Work out the finished part from the listing and answer in its coordinate system (mm). Face numbers are marked on the shaded views. A direction names the side the tool comes from. Coordinates: 2 decimals unless noted, no trailing zeros. Order: outer loops, then holes, each group sorted by start corner. A loop starts at its lowest first (then second) coordinate and runs counter-clockwise, first axis right, second up. Notation, with made-up numbers: (29.25, -30) - (44.25, -30) arc R21 cw to (44.25, -7) - close; hole circle Ø7 at (36, 85.25). An arc over 180 degrees is marked (long way). Use CSV: the item, a comma, the result in double quotes. Start each with the question number.
from build123d import *

# Parameters (mm, degrees)
SKETCH1_R               = 6.5
BOSS_EXTRUDE1_DEPTH     = 17.5
SKETCH2_R               = 8.62249149
SKETCH2_R_2             = 5.56
CUT_EXTRUDE1_DEPTH      = 8
CUT_EXTRUDE2_DEPTH      = 20.767397401
CUT_EXTRUDE2_DEPTH_BACK = 20.767397401
SKETCH4_R               = 3
SKETCH5_R               = 8
SKETCH5_R_2             = 3.869185068
BOSS_EXTRUDE2_DEPTH     = 1
SKETCH6_R               = 8
SKETCH6_R_2             = 3
BOSS_EXTRUDE3_DEPTH     = 3.2


with BuildPart() as part:
    # Sketch1 → Boss-Extrude1 (new body)
    with BuildSketch(Plane(origin=(0, 0, 0), x_dir=(1, 0, 0), z_dir=(0, 1, 0))):
        with Locations(Location((0, 0, 0), (0, 0, 270))):
            Circle(SKETCH1_R)
    extrude(amount=BOSS_EXTRUDE1_DEPTH)

    # Sketch2 → Cut-Extrude1 (cut)
    with BuildSketch(Plane(origin=(0, 11.2, 0), x_dir=(1, 0, 0), z_dir=(0, 1, 0))):
        Circle(SKETCH2_R)
        with Locations(Location((0, 0, 0), (0, 0, 270))):
            Circle(SKETCH2_R_2, mode=Mode.SUBTRACT)
    extrude(amount=-CUT_EXTRUDE1_DEPTH, mode=Mode.SUBTRACT)

    # Sketch4 → Cut-Extrude2 (cut, two sides: drawn at the far end of the back side and taken through both)
    with BuildSketch(Plane(origin=(0, 17.5, 0), x_dir=(1, 0, 0), z_dir=(0, 1, 0)).offset(-CUT_EXTRUDE2_DEPTH_BACK)):
        with Locations(Location((0, 0, 0), (0, 0, 270))):
            Circle(SKETCH4_R)
    extrude(amount=CUT_EXTRUDE2_DEPTH + CUT_EXTRUDE2_DEPTH_BACK, mode=Mode.SUBTRACT)

    # Sketch5 → Boss-Extrude2 (add)
    with BuildSketch(Plane(origin=(0, 11.2, 0), x_dir=(1, 0, 0), z_dir=(0, 1, 0))):
        with Locations(Location((0, 0, 0), (0, 0, 270))):
            Circle(SKETCH5_R)
        Circle(SKETCH5_R_2, mode=Mode.SUBTRACT)
    extrude(amount=BOSS_EXTRUDE2_DEPTH)

    # Sketch6 → Boss-Extrude3 (add)
    with BuildSketch(Plane(origin=(0, 0, 0), x_dir=(1, 0, 0), z_dir=(0, 1, 0))):
        with Locations(Location((0, 0, 0), (0, 0, 270))):
            Circle(SKETCH6_R)
        with Locations(Location((0, 0, 0), (0, 0, 270))):
            Circle(SKETCH6_R_2, mode=Mode.SUBTRACT)
    extrude(amount=BOSS_EXTRUDE3_DEPTH)


solid = part.part
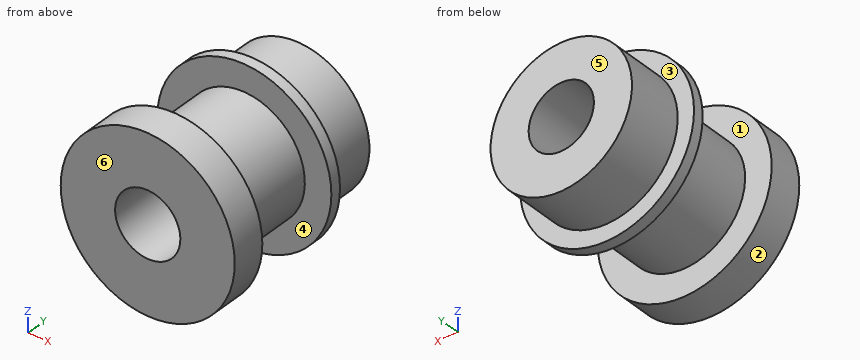
1) For a pull along Y with two mould halves and no side action, classify the marked faces 4, 5 and 6 as +Y half, -Y half, draft (parallel to the pull), parting line (faces both ways), or undercut.
2) The part is cut by section D-D on z = 3.5. Determine the outline of the cut face in (x, y), plus the area to 3 significant figures.
3) The part is cut by section A-A on x = 0. Determine the outline of the cut face in (y, z), plus the area to 3 significant figures.
4) Flat-ended cylindrical pins translate along their axes: P1, Ø6, axis at x = 5, y = 3, coming from the -Z side; P2, Ø5, axis at y = 7.5, z = -4, coming from the +X side; P3, Ø4, axis at y = 15.5, z = -3, coming from the +X side. Find the tip coordinate at first contact, or state that the pin passes through.
5) The part is cut by section C-C on y = 1.5. Determine the outline of the cut face in (x, z), plus the area to 3 significant figures.
6) The part is cut by section B-B on z = 0. Determine the outline of the cut face in (x, y), plus the area to 3 significant figures.
7) For the marked faces 1, 2 and 3, determine the directions among +Z, -Z, +X, -X, +Y, -Y from which every point of the face is accessible in a straight line to the end or side of a thin tool.
8) Straight lines are drawn through the part: line 1 (X direction, y = 4.5, z = 0); line 2 (Y direction, x = 6, z = 1.25); line 3 (Y direction, x = -3.5, z = 6). For each, find the intervals that lie inside material, in ascending order. Write a range as [from, to].
Answer key:
1,face 4,"undercut"
1,face 5,"+Y half"
1,face 6,"-Y half"
2,outline,"(-7.19, 0) - (7.19, 0) - (7.19, 3.2) - (4.32, 3.2) - (4.32, 11.2) - (7.19, 11.2) - (7.19, 12.2) - (5.48, 12.2) - (5.48, 17.5) - (-5.48, 17.5) - (-5.48, 12.2) - (-7.19, 12.2) - (-7.19, 11.2) - (-4.32, 11.2) - (-4.32, 3.2) - (-7.19, 3.2) - close"
2,area,"188 mm^2"
3,outline,"(0, -8) - (3.2, -8) - (3.2, -5.56) - (11.2, -5.56) - (11.2, -8) - (12.2, -8) - (12.2, -6.5) - (17.5, -6.5) - (17.5, -3) - (0, -3) - close; (0, 3) - (17.5, 3) - (17.5, 6.5) - (12.2, 6.5) - (12.2, 8) - (11.2, 8) - (11.2, 5.56) - (3.2, 5.56) - (3.2, 8) - (0, 8) - close"
3,area,"120 mm^2"
4,P1,"z = -7.75"
4,P2,"x = 5.35"
4,P3,"x = 6.42"
5,outline,"circle Ø16 at (0, 0); hole circle Ø6 at (0, 0)"
5,area,"173 mm^2"
6,outline,"(-8, 0) - (-3, 0) - (-3, 17.5) - (-6.5, 17.5) - (-6.5, 12.2) - (-8, 12.2) - (-8, 11.2) - (-5.56, 11.2) - (-5.56, 3.2) - (-8, 3.2) - close; (3, 0) - (8, 0) - (8, 3.2) - (5.56, 3.2) - (5.56, 11.2) - (8, 11.2) - (8, 12.2) - (6.5, 12.2) - (6.5, 17.5) - (3, 17.5) - close"
6,area,"120 mm^2"
7,face 1,"none"
7,face 2,"+Y, -Y"
7,face 3,"+Y"
8,line 1,"[-5.56, -3], [3, 5.56]"
8,line 2,"[0, 3.2], [11.2, 17.5]"
8,line 3,"[0, 3.2], [11.2, 12.2]"
